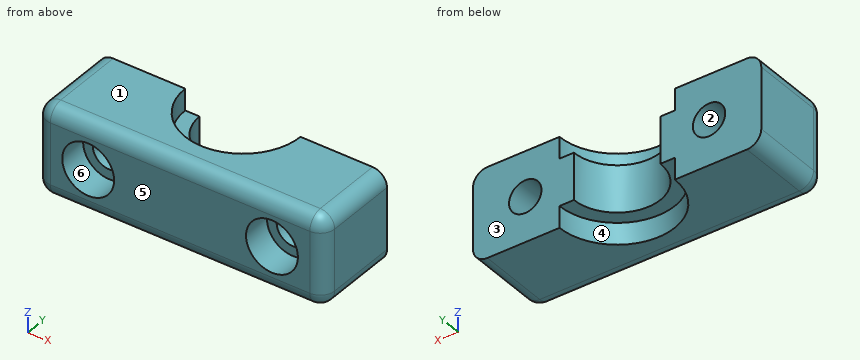
```python
from build123d import *

# Parameters (mm, degrees)
F0_W          = 40
F0_H          = 12.5
F0_R          = 2.25
F1_DEPTH      = 6
F1_DEPTH_BACK = 6
F2_R          = 3.6
F3_DEPTH      = 4
F4_R          = 2
F6_DEPTH      = 6.25
F6_DEPTH_BACK = 6.25
F7_R          = 8
F8_DEPTH      = 3
F9_R          = 8
F10_DEPTH     = 3


with BuildPart() as f1:
    # F0 (on Front) → F1 (new body, two sides)
    with BuildSketch(Plane.XZ) as f1_sk:
        Rectangle(F0_W, F0_H)
        with Locations((-12.75, 0)):
            Circle(F0_R, mode=Mode.SUBTRACT)
        with Locations((12.75, 0)):
            Circle(F0_R, mode=Mode.SUBTRACT)
    extrude(amount=F1_DEPTH)
    extrude(f1_sk.sketch, amount=-F1_DEPTH_BACK)

    # F2 (on face) → F3 (cut)
    with BuildSketch(Plane.XZ.offset(6)):
        with Locations((-12.75, 0)):
            Circle(F2_R)
        with Locations((12.75, 0)):
            Circle(F2_R)
    extrude(amount=-F3_DEPTH, mode=Mode.SUBTRACT)

    # F4
    f4_edges = [f1.edges().sort_by_distance(p)[0] for p in [
        (-20, 0, 6.25),
        (-20, 0, -6.25),
        (20, 0, 6.25),
        (20, 0, -6.25),
        (20, -6, 0),
        (0, -6, 6.25),
        (0, -6, -6.25),
        (-20, -6, 0),
    ]]
    fillet(f4_edges, radius=F4_R)

    # F5 (on Top) → F6 (cut, two sides)
    with BuildSketch(Plane.XY) as f6_sk:
        with BuildLine():
            Line((6, 6), (-6, 6))
            ThreePointArc((-6, 6), (0, 0), (6, 6))
        make_face()
    extrude(amount=-F6_DEPTH, mode=Mode.SUBTRACT)
    extrude(f6_sk.sketch, amount=F6_DEPTH_BACK, mode=Mode.SUBTRACT)

    # F7 (on face) → F8 (cut)
    with BuildSketch(Plane.XY.offset(6.25)):
        with Locations((0, 6)):
            Circle(F7_R)
    extrude(amount=-F8_DEPTH, mode=Mode.SUBTRACT)

    # F9 (on face) → F10 (cut)
    with BuildSketch(Plane(origin=(0, 0, -6.25), x_dir=(1, 0, 0), z_dir=(0, 0, -1))):
        with Locations((0, -6)):
            Circle(F9_R)
    extrude(amount=-F10_DEPTH, mode=Mode.SUBTRACT)


solid = f1.part
```
Could you check a few things on this model? Use its own coordinates, in mm. Face numbers are marked on the shaded views. A direction names the side the tool comes from. Give positions to 0.01 mm unless a question says otherwise; leave off trailing zeros. Loops run counter-clockwise (first coordinate to the right, second up) from the corner with the lowest first, then second, coordinate; pieces in that order, holes last. Notation, with made-up numbers: (56, 34) - (106, 34) arc R17 cw to (106, 62) - close; hole circle Ø4 at (52, 55). An arc over 180 degrees is marked (long way). Answer in a Markdown table with one row per item. Add a question column.
Q1. Which directions (+Z, -Z, +X, -X, +Y, -Y) give clear straight access to the entire face, cutting with the end or side of a thin tool? Please do the marked faces 4, 5 and 6.
Q2. If we section it at B-B (y = 5): List the corners of the cut face in (x, z) for me, plus the area to 3 significant figures.
Q3. If we section it at D-D (x = 0): List the corners of the cut face in (y, z) for me, plus the area to 3 significant figures.
Q4. If we section it at A-A (x = -12.75): List the corners of the cut face in (y, z) for me.
Q5. Please list where these lines run through material, in increasing order: L1, parallel to X at y = 2, z = 0; L2, parallel to X at y = 5.25, z = 1.75; L3, parallel to X at y = -4.75, z = -1.5. Write a range as from..to.
Q6. We'd pull the mould along Z, two halves only. Please class the marked faces 1, 2 and 3: +Z half, -Z half, draft (parallel to the pull), parting line (faces both ways), or undercut.
Q7. For pin 1 (6 mm diameter, centred on x = -14, z = 5, fed in from -Y); pin 2 (4 mm diameter, centred on x = 2, y = 1.5, fed in from -Z); pin 3 (3.5 mm diameter, centred on x = 13, z = -1.5, fed in from -Y), each with a flat end and sliding along its axis, tell me the tip position at first contact or that it passes through.
Q8. If we section it at C-C (z = 1.25): List the corners of the cut face in (x, y) for me, plus the area to 3 significant figures.
The answers:
| question | item | result |
|---|---|---|
| 1 | face 4 | -Z, +Y |
| 1 | face 5 | +Z, -Z, +X, -X, -Y |
| 1 | face 6 | -Y |
| 2 | outline | (-20, -4.25) arc R2 ccw to (-18, -6.25) - (-7.94, -6.25) - (-7.94, -3.25) - (-5.92, -3.25) - (-5.92, 3.25) - (-7.94, 3.25) - (-7.94, 6.25) - (-18, 6.25) arc R2 ccw to (-20, 4.25) - close; (5.92, -3.25) - (7.94, -3.25) - (7.94, -6.25) - (18, -6.25) arc R2 ccw to (20, -4.25) - (20, 4.25) arc R2 ccw to (18, 6.25) - (7.94, 6.25) - (7.94, 3.25) - (5.92, 3.25) - close; hole circle Ø4.5 at (-12.75, 0); hole circle Ø4.5 at (12.75, 0) |
| 2 | area | 293 mm^2 |
| 3 | outline | (-6, -4.25) arc R2 ccw to (-4, -6.25) - (-2, -6.25) - (-2, -3.25) - (0, -3.25) - (0, 3.25) - (-2, 3.25) - (-2, 6.25) - (-4, 6.25) arc R2 ccw to (-6, 4.25) - close |
| 3 | area | 61.3 mm^2 |
| 4 | outline | (-6, -4.25) arc R2 ccw to (-4, -6.25) - (6, -6.25) - (6, -2.25) - (-2, -2.25) - (-2, -3.6) - (-6, -3.6) - close; (-6, 3.6) - (-2, 3.6) - (-2, 2.25) - (6, 2.25) - (6, 6.25) - (-4, 6.25) arc R2 ccw to (-6, 4.25) - close |
| 5 | L1 | x = -20..-15, -10.5..-4.47, 4.47..10.5, 15..20 |
| 5 | L2 | x = -20..-14.16, -11.34..-5.95, 5.95..11.34, 14.16..20 |
| 5 | L3 | x = -19.85..-16.02, -9.48..9.48, 16.02..19.85 |
| 6 | face 1 | +Z half |
| 6 | face 2 | undercut |
| 6 | face 3 | draft |
| 7 | pin 1 | stops at y = -6 |
| 7 | pin 2 | stops at z = -3.25 |
| 7 | pin 3 | stops at y = -2 |
| 8 | outline | (-20, -4) arc R2 ccw to (-18, -6) - (-16.13, -6) - (-16.13, -2) - (-14.62, -2) - (-14.62, 6) - (-20, 6) - close; (-10.88, -2) - (-9.37, -2) - (-9.37, -6) - (9.37, -6) - (9.37, -2) - (10.88, -2) - (10.88, 6) - (6, 6) arc R6 cw to (-6, 6) - (-10.88, 6) - close; (14.62, -2) - (16.13, -2) - (16.13, -6) - (18, -6) arc R2 ccw to (20, -4) - (20, 6) - (14.62, 6) - close |
| 8 | area | 308 mm^2 |
